Build history of the part. All positions in model axes, mm. A direction names the side the tool comes from. Coordinates: 2 decimals unless noted, no trailing zeros. Loops run counter-clockwise (first coordinate to the right, second up) from the corner with the lowest first, then second, coordinate; pieces in that order, holes last.
(1) Tool access for faces 1 (the face through (0, 0, 4)), 2 (the face through (0, 5.08, 4)): list every direction of +Z, -Z, +X, -X, +Y, -Y with a clear straight run to the whole face (end or side of a thin tool).
(2) Slice it at A-A (y = 8.25). Give the cut face in (x, z), and give its area (3 significant figures).
(3) Slice it at B-B (z = 225). Give the cut face in (x, y) (3 decimals).
(4) Wall check: L1, parallel to X at y = 9.75, z = -125.5; L2, parallel to X at y = 9, z = -106; L3, parallel to Y at x = 13, z = 120.5. Give the ranges that are in metal, low to high.
(5) Flat gauge pins, fed straight in: P1, Ø5, axis at x = 0, z = 241.3, coming from the +Y side; P2, Ø1.5, axis at x = 12, z = -207, coming from the +Y side; P3, Ø4, axis at y = 6, z = 225, coming from the +X side; P4, Ø1.3, axis at y = 1.5, z = -137, coming from the -X side. Where does each tip first touch, or does it go through?
from build123d import *

# Parameters (mm, degrees)
BOSS_EXTRUDE1_DEPTH = 304.8
SKETCH2_R           = 3.2766
CUT_EXTRUDE2_DEPTH  = 306.95635975
SKETCH4_R           = 3.2766
CUT_EXTRUDE4_DEPTH  = 25.4
SKETCH5_R           = 3.2766
CUT_EXTRUDE5_DEPTH  = 25.4
SKETCH6_R           = 3.2766
CUT_EXTRUDE8_DEPTH  = 25.4


with BuildPart() as part:
    # Sketch1 → Boss-Extrude1 (new, symmetric)
    with BuildSketch(Plane.XY):
        with BuildLine():
            Line((-14.605, 5.08), (14.605, 5.08))
            Line((14.605, 5.08), (16.174141854, 5.985944472))
            ThreePointArc((16.174141854, 5.985944472), (22.730946929, 13.208062038), (19.05, 4.174717993))
            Line((19.05, 4.174717993), (19.05, 0))
            Line((19.05, 0), (-19.05, 0))
            Line((-19.05, 0), (-19.05, 4.174717993))
            ThreePointArc((-19.05, 4.174717993), (-22.730946929, 13.208062038), (-16.174141854, 5.985944472))
            Line((-16.174141854, 5.985944472), (-14.605, 5.08))
        make_face()
    extrude(amount=BOSS_EXTRUDE1_DEPTH, both=True)

    # Sketch2 → Cut-Extrude2 (cut, through all)
    with BuildSketch(Plane(origin=(0, 5.08, 0), x_dir=(1, 0, 0), z_dir=(0, 1, 0))):
        with Locations(Location((0, -292.1, 0), (0, 0, 270))):
            Circle(SKETCH2_R)
    extrude(amount=-CUT_EXTRUDE2_DEPTH, mode=Mode.SUBTRACT)

    # Sketch4 → Cut-Extrude4 (cut)
    with BuildSketch(Plane(origin=(0, 5.08, 0), x_dir=(1, 0, 0), z_dir=(0, 1, 0))):
        with Locations(Location((0, -241.3, 0), (0, 0, 270))):
            Circle(SKETCH4_R)
        with Locations(Location((0, -120.65, 0), (0, 0, 270))):
            Circle(SKETCH4_R)
        with Locations(Location((0, 0, 0), (0, 0, 270))):
            Circle(SKETCH4_R)
        with Locations(Location((0, 120.65, 0), (0, 0, 270))):
            Circle(SKETCH4_R)
        with Locations(Location((0, 241.3, 0), (0, 0, 270))):
            Circle(SKETCH4_R)
    extrude(amount=-CUT_EXTRUDE4_DEPTH, mode=Mode.SUBTRACT)

    # Sketch5 → Cut-Extrude5 (cut)
    with BuildSketch(Plane(origin=(0, 5.08, 0), x_dir=(1, 0, 0), z_dir=(0, 1, 0))):
        with Locations(Location((0, 292.1, 0), (0, 0, 270))):
            Circle(SKETCH5_R)
    extrude(amount=-CUT_EXTRUDE5_DEPTH, mode=Mode.SUBTRACT)

    # Sketch6 → Cut-Extrude8 (cut)
    with BuildSketch(Plane(origin=(0, 5.08, 0), x_dir=(1, 0, 0), z_dir=(0, 1, 0))):
        with Locations(Location((0, 264.16, 0), (0, 0, 270))):
            Circle(SKETCH6_R)
    extrude(amount=-CUT_EXTRUDE8_DEPTH, mode=Mode.SUBTRACT)


solid = part.part
Response values:
1. face 1: +Z, -Z, +X, -X, -Y
1. face 2: +Z, -Z, +Y
2. outline: (-24.98, -304.8) - (-15.2, -304.8) - (-15.2, 304.8) - (-24.98, 304.8) - close; (15.2, -304.8) - (24.98, -304.8) - (24.98, 304.8) - (15.2, 304.8) - close
2. area: 11,900 mm2
3. outline: (-19.05, 0) - (19.05, 0) - (19.05, 4.175) arc R4.953 ccw (long way) to (16.174, 5.986) - (14.605, 5.08) - (-14.605, 5.08) - (-16.174, 5.986) arc R4.953 ccw (long way) to (-19.05, 4.175) - close
4. L1: x = -24.99 to -15.19, 15.19 to 24.99
4. L2: x = -25.04 to -15.14, 15.14 to 25.04
4. L3: y = 0 to 5.08
5. P1: passes through
5. P2: stops at y = 5.08
5. P3: stops at x = 24.94
5. P4: stops at x = -19.05
